```python
from build123d import *

# Parameters (mm, degrees)
F0_W      = 279.4
F0_H      = 406.4
F1_DEPTH  = 19.05
F2_R      = 19.05
F4_DEPTH  = 19.05
F6_DEPTH  = 19.05
F7_W      = 19.05
F7_H      = 38.1
F8_DEPTH  = 19.05
F10_DEPTH = 19.05
F11_R     = 3.175


with BuildPart() as f1:
    # F0 (on Front) → F1 (new body)
    with BuildSketch(Plane.XZ):
        with Locations((139.7, 203.2)):
            Rectangle(F0_W, F0_H)
    extrude(amount=F1_DEPTH)

    # F2
    f2_edges = [f1.edges().sort_by_distance(p)[0] for p in [
        (0, -9.525, 406.4),
        (279.4, -9.525, 406.4),
    ]]
    fillet(f2_edges, radius=F2_R)

    # F3 (on face) → F4 (cut)
    with BuildSketch(Plane.XZ.offset(19.05)):
        Polygon((0, 0), (38.1, 0), (38.1, 19.05), (57.15, 19.05), (57.15, 38.1), (38.1, 38.1), (38.1, 57.15), (19.05, 57.15), (19.05, 38.1), (0, 38.1), align=None)
        Polygon((241.3, 19.05), (241.3, 0), (279.4, 0), (279.4, 38.1), (260.35, 38.1), (260.35, 57.15), (241.3, 57.15), (241.3, 38.1), (222.25, 38.1), (222.25, 19.05), align=None)
    extrude(amount=-F4_DEPTH, mode=Mode.SUBTRACT)

    # F5 (on face) → F6 (cut)
    with BuildSketch(Plane.XZ.offset(19.05)):
        with BuildLine():
            Line((19.05, 50.8), (19.05, 57.15))
            ThreePointArc((19.05, 57.15), (15.875, 53.975), (19.05, 50.8))
        make_face()
        with BuildLine():
            ThreePointArc((38.1, 50.8), (41.275, 53.975), (38.1, 57.15))
            Line((38.1, 57.15), (38.1, 50.8))
        make_face()
        with BuildLine():
            Line((50.8, 38.1), (57.15, 38.1))
            ThreePointArc((57.15, 38.1), (53.975, 41.275), (50.8, 38.1))
        make_face()
        with BuildLine():
            ThreePointArc((50.8, 19.05), (53.975, 15.875), (57.15, 19.05))
            Line((57.15, 19.05), (50.8, 19.05))
        make_face()
        with BuildLine():
            Line((228.6, 19.05), (222.25, 19.05))
            ThreePointArc((222.25, 19.05), (225.425, 15.875), (228.6, 19.05))
        make_face()
        with BuildLine():
            ThreePointArc((228.6, 38.1), (225.425, 41.275), (222.25, 38.1))
            Line((222.25, 38.1), (228.6, 38.1))
        make_face()
        with BuildLine():
            Line((241.3, 50.8), (241.3, 57.15))
            ThreePointArc((241.3, 57.15), (238.125, 53.975), (241.3, 50.8))
        make_face()
        with BuildLine():
            ThreePointArc((260.35, 50.8), (263.525, 53.975), (260.35, 57.15))
            Line((260.35, 57.15), (260.35, 50.8))
        make_face()
    extrude(amount=-F6_DEPTH, mode=Mode.SUBTRACT)

    # F7 (on face) → F8 (cut)
    with BuildSketch(Plane.XZ.offset(19.05)):
        with Locations((28.575, 368.3)):
            Rectangle(F7_W, F7_H)
        with Locations((250.825, 368.3)):
            Rectangle(F7_W, F7_H)
    extrude(amount=-F8_DEPTH, mode=Mode.SUBTRACT)

    # F9 (on face) → F10 (cut)
    with BuildSketch(Plane.XZ.offset(19.05)):
        with BuildLine():
            Line((19.05, 381), (19.05, 387.35))
            ThreePointArc((19.05, 387.35), (15.875, 384.175), (19.05, 381))
        make_face()
        with BuildLine():
            ThreePointArc((19.05, 355.6), (15.875, 352.425), (19.05, 349.25))
            Line((19.05, 349.25), (19.05, 355.6))
        make_face()
        with BuildLine():
            Line((38.1, 355.6), (38.1, 349.25))
            ThreePointArc((38.1, 349.25), (41.275, 352.425), (38.1, 355.6))
        make_face()
        with BuildLine():
            ThreePointArc((38.1, 381), (41.275, 384.175), (38.1, 387.35))
            Line((38.1, 387.35), (38.1, 381))
        make_face()
        with BuildLine():
            Line((241.3, 381), (241.3, 387.35))
            ThreePointArc((241.3, 387.35), (238.125, 384.175), (241.3, 381))
        make_face()
        with BuildLine():
            ThreePointArc((260.35, 381), (263.525, 384.175), (260.35, 387.35))
            Line((260.35, 387.35), (260.35, 381))
        make_face()
        with BuildLine():
            ThreePointArc((241.3, 355.6), (238.125, 352.425), (241.3, 349.25))
            Line((241.3, 349.25), (241.3, 355.6))
        make_face()
        with BuildLine():
            Line((260.35, 355.6), (260.35, 349.25))
            ThreePointArc((260.35, 349.25), (263.525, 352.425), (260.35, 355.6))
        make_face()
    extrude(amount=-F10_DEPTH, mode=Mode.SUBTRACT)

    # F11
    f11_edges = [f1.edges().sort_by_distance(p)[0] for p in [
        (0, -9.525, 38.1),
        (19.05, -9.525, 38.1),
        (38.1, -9.525, 38.1),
        (38.1, -9.525, 0),
        (241.3, -9.525, 0),
        (241.3, -9.525, 19.05),
        (241.3, -9.525, 38.1),
        (260.35, -9.525, 38.1),
        (279.4, -9.525, 38.1),
        (38.1, -9.525, 19.05),
    ]]
    fillet(f11_edges, radius=F11_R)


solid = f1.part
```
Could you check a few things on this model? Use its own coordinates, in mm. A direction names the side the tool comes from. Give positions to 0.01 mm unless a question says otherwise; leave off trailing zeros. Write each loop counter-clockwise with the first axis right and the second up, starting at its lowest first coordinate (ties: lowest second). Pieces come first, ordered by that corner, then holes. Notation, with made-up numbers: (-3, 58.25) -> (17, 58.25) arc R14 cw to (17, 85.25) -> close; hole circle Ø5 at (-19.75, -39). An arc over 180 degrees is marked (long way). Write each question's results on one line, items separated by ' | '.
1. I need wall thicknesses on L1, parallel to X at y = -10.5, z = 46.5; L2, parallel to Z at x = 239, y = -17.25; L3, parallel to X at y = -4.5, z = 29. Which ranges of each line are inside material? Lowest first, please.
Check sheet entries:
L1: x = 0 to 19.05, 38.1 to 241.3, 260.35 to 279.4 | L2: z = 0.12 to 18.93, 38.22 to 51.79, 56.16 to 350.24, 354.61 to 381.99, 386.36 to 406.4 | L3: x = 57.15 to 222.25
2. I want a section at A-A, the plane x = 252.5. Write out the boundary of the cut face in (y, z), then the cut area to 3 significant figures.
Check sheet entries:
outline: (-19.05, 57.15) -> (0, 57.15) -> (0, 349.25) -> (-19.05, 349.25) -> close; (-19.05, 387.35) -> (0, 387.35) -> (0, 406.4) -> (-19.05, 406.4) -> close | area: 5,930 mm²
3. I want a section at B-B, the plane y = -9.5. Count the separate pieces of the cut face and the enclosed holes in it, then the cut area to 3 significant figures.
Check sheet entries:
separate pieces: 1 | enclosed holes: 2 | area: 107,000 mm²
4. Will these pins go through, and if not, where does the flat tip stop? pin 1 Ø9.5 at (y, z) = (-8.5, 29.5) entering from -X; pin 2 Ø5.5 at (x, y) = (250, -7.5) entering from -Z; pin 3 Ø10 at (x, y) = (270, -13.5) entering from -Z.
Check sheet entries:
pin 1: stops at x = 57.15 | pin 2: stops at z = 57.15 | pin 3: stops at z = 38.1
5. If we mould it in two halves opening along Z, with no side actions, what happens to faces 1 (the flat face through (138, -9, 0)), 2 (the flat face through (0, -9, 212)), 3 (the cylindrical face through (5.43, -9.66, 400.67)), 4 (the flat face through (38.1, -10, 368))? For each: released by +Z, released by -Z, zero draft, split by the parting line, or undercut.
Check sheet entries:
face 1: released by -Z | face 2: zero draft | face 3: released by +Z | face 4: undercut
6. On a 3-axis mill with a long thin cutter (end or side, diameter ignored), from which of +Z, -Z, +X, -X, +Y, -Y can I reach the whole of each face in a straight line? I mean faces 5 (the flat face through (38.1, -10, 46)), 6 (the flat face through (46, -10, 19.05)), 7 (the flat face through (241.3, -10, 10)), 8 (the flat face through (251, -10, 349.25)). Say none if no direction works.
Check sheet entries:
face 5: -Z, +Y, -Y | face 6: -X, +Y, -Y | face 7: -Z, +X, +Y, -Y | face 8: +Y, -Y
